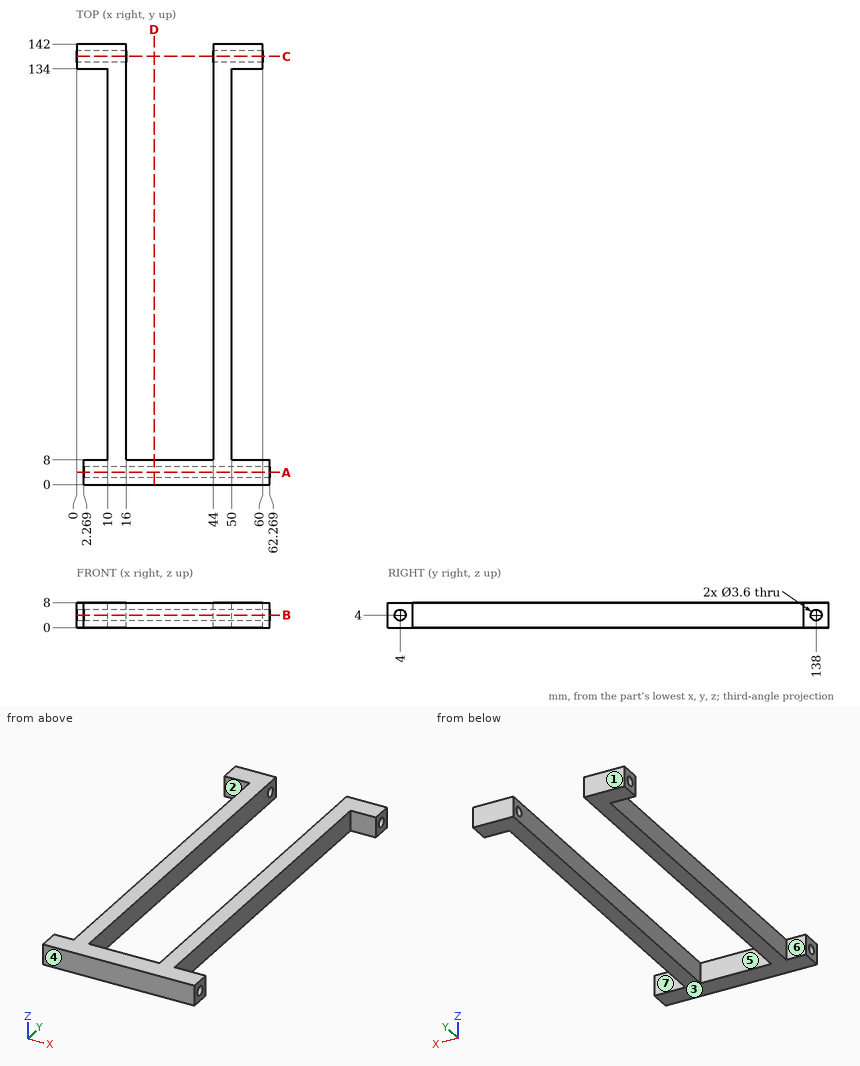
Geometry: see drawing. Coordinates: mm, zero at the bounding-box minimum. A direction names the side the tool comes from. Coordinates: 2 decimals unless noted, no trailing zeros. Order: outer loops, then holes, each group sorted by start corner. A loop starts at its lowest first (then second) coordinate and runs counter-clockwise, first axis right, second up. Notation, with made-up numbers: (-24.5, 13.25) -> (-7.5, 13.25) arc R8 cw to (-7.5, 22.25) -> close; hole circle Ø2 at (52, -28). An arc over 180 degrees is marked (long way). Write each question's results on one line, items separated by ' | '. Start each with the question number.
1) First-contact query: pin 1 (4 mm diameter, centred on y = 49.5, z = 3.5, fed in from +X); pin 2 (1.5 mm diameter, centred on y = 62, z = 4.5, fed in from -X); pin 3 (2.5 mm diameter, centred on y = 137, z = 3.5, fed in from +X); pin 4 (3 mm diameter, centred on y = 4, z = 4, fed in from -X). Flat tips, straight axial feed; report the tip coordinate or a pass-through.
2) Material intervals for line 1 along Y through (x, z) = (6.25, 4); line 2 along Y through (x, z) = (46, 4); line 3 along X through (y, z) = (58.5, 3.25), sorted ascending.
3) Cut plane B-B, the plane z = 4. Output: boundary loops of the cut face in (x, y).
4) Cut plane D-D, the plane x = 25. Output: boundary loops of the cut face in (y, z), and give its area (3 significant figures).
5) Cut plane C-C, the plane y = 138. Output: boundary loops of the cut face in (x, z).
6) Cut plane A-A, the plane y = 4. Output: boundary loops of the cut face in (x, z), and give its area (3 significant figures).
7) Mould query, pull axis Y, two halves, no side actions, for the marked faces 1, 2, 3 and 4. Classes: released by +Y, released by -Y, zero draft, split by the parting line, or undercut.
8) Set-up query: the marked faces 5, 6 and 7. Return all of +Z, -Z, +X, -X, +Y, -Y with unobstructed straight access to the full face (end or side cutting, diameter ignored); none if empty.
Checks:
1) pin 1: x = 50 | pin 2: x = 10 | pin 3: x = 60 | pin 4: through
2) line 1: 0 to 2.2, 5.8 to 8, 134 to 136.2, 139.8 to 142 | line 2: 0 to 2.2, 5.8 to 136.2, 139.8 to 142 | line 3: 10 to 16, 44 to 50
3) outline: (0, 134) -> (10, 134) -> (10, 8) -> (2.27, 8) -> (2.27, 5.8) -> (62.27, 5.8) -> (62.27, 8) -> (50, 8) -> (50, 134) -> (60, 134) -> (60, 136.2) -> (44, 136.2) -> (44, 8) -> (16, 8) -> (16, 136.2) -> (0, 136.2) -> close; (0, 139.8) -> (16, 139.8) -> (16, 142) -> (0, 142) -> close; (2.27, 0) -> (62.27, 0) -> (62.27, 2.2) -> (2.27, 2.2) -> close; (44, 139.8) -> (60, 139.8) -> (60, 142) -> (44, 142) -> close
4) outline: (0, 0) -> (8, 0) -> (8, 8) -> (0, 8) -> close; hole circle Ø3.6 at (4, 4) | area: 53.8 mm^2
5) outline: (0, 0) -> (16, 0) -> (16, 2.2) -> (0, 2.2) -> close; (0, 5.8) -> (16, 5.8) -> (16, 8) -> (0, 8) -> close; (44, 0) -> (60, 0) -> (60, 2.2) -> (44, 2.2) -> close; (44, 5.8) -> (60, 5.8) -> (60, 8) -> (44, 8) -> close
6) outline: (2.27, 0) -> (62.27, 0) -> (62.27, 2.2) -> (2.27, 2.2) -> close; (2.27, 5.8) -> (62.27, 5.8) -> (62.27, 8) -> (2.27, 8) -> close | area: 264 mm^2
7) face 1: released by +Y | face 2: undercut | face 3: zero draft | face 4: released by -Y
8) face 5: +Z, -Z, +Y | face 6: +Z, -Z, -X | face 7: +Z, -Z, +X
